Design review of the part built by this model. Coordinates are the model's own, in mm. A direction names the side the tool comes from. Give positions to 0.01 mm unless a question says otherwise; leave off trailing zeros. Order: outer loops, then holes, each group sorted by start corner. A loop starts at its lowest first (then second) coordinate and runs counter-clockwise, first axis right, second up. Notation, with made-up numbers: (30.25, 86) -> (48.25, 86) arc R25 ccw to (48.25, 100) -> close; hole circle Ø7 at (-4, 39). An arc over 180 degrees is marked (long way). One line per item, written item: value. Start each with the question number.
1) Consider section B-B (y = -7.5). State the section outline as (x, z) points, plus the area to 3 significant figures.
2) Tool access review of faces 5 (the face through (34.5, 9, 1)), 6 (the face through (-35, 7.5, 1)), 7 (the face through (12, 7, 1)), 8 (the face through (35, 1.5, 1)): name each direction out of +Z, -Z, +X, -X, +Y, -Y from which nothing blocks a thin tool from reaching the whole face with its end or side.
3) For pin 1 (0.6 mm diameter, centred on x = 35.5, z = 1, fed in from -Y); pin 2 (0.6 mm diameter, centred on x = -35, z = 1, fed in from +Y); pin 3 (7 mm diameter, centred on x = -25, y = -5.5, fed in from +Z), all flat-tipped, find the tip position at first contact; note any pin that passes through.
4) Consider section A-A (x = 15). State the section outline as (y, z) points.
5) Consider section D-D (x = 25). State the section outline as (y, z) points.
6) Consider section C-C (z = 1.2). State how many separate pieces and enclosed holes the cut face has, plus the area to 3 significant figures.
7) The part is to be moulded in two halves that separate along Y. For faces 1 (the face through (37.5, 4, 1)), 2 (the face through (36, 7.5, 1)), 3 (the face through (17, -6, 1)), 4 (the face through (-28.2, -7.9, 1)), say which applies: released by +Y, released by -Y, zero draft, split by the parting line, or undercut.
8) Wall thickness on line 1 along X through (y, z) = (2.75, 0.55); line 2 along X through (y, z) = (11, 0.9); line 3 along Y through (x, z) = (-25, 0.95): over which ranges is each line inside the solid? List them lowest first. Write a range as from..to.
from build123d import *

# Parameters (mm, degrees)
ESBO_O1_R                = 4
ESBO_O1_R_2              = 2.5
RESSALTO_EXTRUS_O1_DEPTH = 2


with BuildPart() as part:
    # Esboço1 → Ressalto-extrusão1 (new body)
    with BuildSketch(Plane.XY):
        with BuildLine():
            Line((-34.5, 1.5), (-34.5, -6.5))
            ThreePointArc((-34.5, -6.5), (-32.742640687, -10.742640687), (-28.5, -12.5))
            Line((-28.5, -12.5), (28.5, -12.5))
            ThreePointArc((28.5, -12.5), (32.742640687, -10.742640687), (34.5, -6.5))
            Line((34.5, -6.5), (34.5, 1.5))
            Line((34.5, 1.5), (36.5, 1.5))
            ThreePointArc((36.5, 1.5), (37.207106781, 1.792893219), (37.5, 2.5))
            Line((37.5, 2.5), (37.5, 6.5))
            ThreePointArc((37.5, 6.5), (37.207106781, 7.207106781), (36.5, 7.5))
            Line((36.5, 7.5), (34.5, 7.5))
            Line((34.5, 7.5), (34.5, 11.5))
            ThreePointArc((34.5, 11.5), (34.207106781, 12.207106781), (33.5, 12.5))
            Line((33.5, 12.5), (13, 12.5))
            ThreePointArc((13, 12.5), (12.292893219, 12.207106781), (12, 11.5))
            Line((12, 11.5), (12, 1.5))
            ThreePointArc((12, 1.5), (11, 0.5), (10, 1.5))
            Line((10, 1.5), (10, 11.5))
            ThreePointArc((10, 11.5), (9.707106781, 12.207106781), (9, 12.5))
            Line((9, 12.5), (-9, 12.5))
            ThreePointArc((-9, 12.5), (-9.707106781, 12.207106781), (-10, 11.5))
            Line((-10, 11.5), (-10, 1.5))
            ThreePointArc((-10, 1.5), (-11, 0.5), (-12, 1.5))
            Line((-12, 1.5), (-12, 11.5))
            ThreePointArc((-12, 11.5), (-12.292893219, 12.207106781), (-13, 12.5))
            Line((-13, 12.5), (-33.5, 12.5))
            ThreePointArc((-33.5, 12.5), (-34.207106781, 12.207106781), (-34.5, 11.5))
            Line((-34.5, 11.5), (-34.5, 7.5))
            Line((-34.5, 7.5), (-36.5, 7.5))
            ThreePointArc((-36.5, 7.5), (-37.207106781, 7.207106781), (-37.5, 6.5))
            Line((-37.5, 6.5), (-37.5, 2.5))
            ThreePointArc((-37.5, 2.5), (-37.207106781, 1.792893219), (-36.5, 1.5))
            Line((-36.5, 1.5), (-34.5, 1.5))
        make_face()
        with Locations((-25, -5.5)):
            Circle(ESBO_O1_R, mode=Mode.SUBTRACT)
        with Locations((-15, -7.5)):
            Circle(ESBO_O1_R_2, mode=Mode.SUBTRACT)
        with Locations(Location((15, -7.5, 0), (0, 0, 180))):
            Circle(ESBO_O1_R_2, mode=Mode.SUBTRACT)
        with Locations(Location((25, -5.5, 0), (0, 0, 180))):
            Circle(ESBO_O1_R, mode=Mode.SUBTRACT)
    extrude(amount=RESSALTO_EXTRUS_O1_DEPTH)


solid = part.part
Checked values:
1. outline: (-34.42, 0) -> (-28.46, 0) -> (-28.46, 2) -> (-34.42, 2) -> close; (-21.54, 0) -> (-17.5, 0) -> (-17.5, 2) -> (-21.54, 2) -> close; (-12.5, 0) -> (12.5, 0) -> (12.5, 2) -> (-12.5, 2) -> close; (17.5, 0) -> (21.54, 0) -> (21.54, 2) -> (17.5, 2) -> close; (28.46, 0) -> (34.42, 0) -> (34.42, 2) -> (28.46, 2) -> close
1. area: 90.0 mm^2
2. face 5: +Z, -Z, +X, +Y
2. face 6: +Z, -Z, -X, +Y
2. face 7: +Z, -Z, +Y
2. face 8: +Z, -Z, +X, -Y
3. pin 1: stops at y = 1.5
3. pin 2: stops at y = 7.5
3. pin 3: passes through
4. outline: (-12.5, 0) -> (-10, 0) -> (-10, 2) -> (-12.5, 2) -> close; (-5, 0) -> (12.5, 0) -> (12.5, 2) -> (-5, 2) -> close
5. outline: (-12.5, 0) -> (-9.5, 0) -> (-9.5, 2) -> (-12.5, 2) -> close; (-1.5, 0) -> (12.5, 0) -> (12.5, 2) -> (-1.5, 2) -> close
6. separate pieces: 1
6. enclosed holes: 4
6. area: 1,560 mm^2
7. face 1: zero draft
7. face 2: released by +Y
7. face 3: undercut
7. face 4: undercut
8. line 1: x = -37.5..-12, -10..10, 12..37.5
8. line 2: x = -34.5..-12, -10..10, 12..34.5
8. line 3: y = -12.5..-9.5, -1.5..12.5
